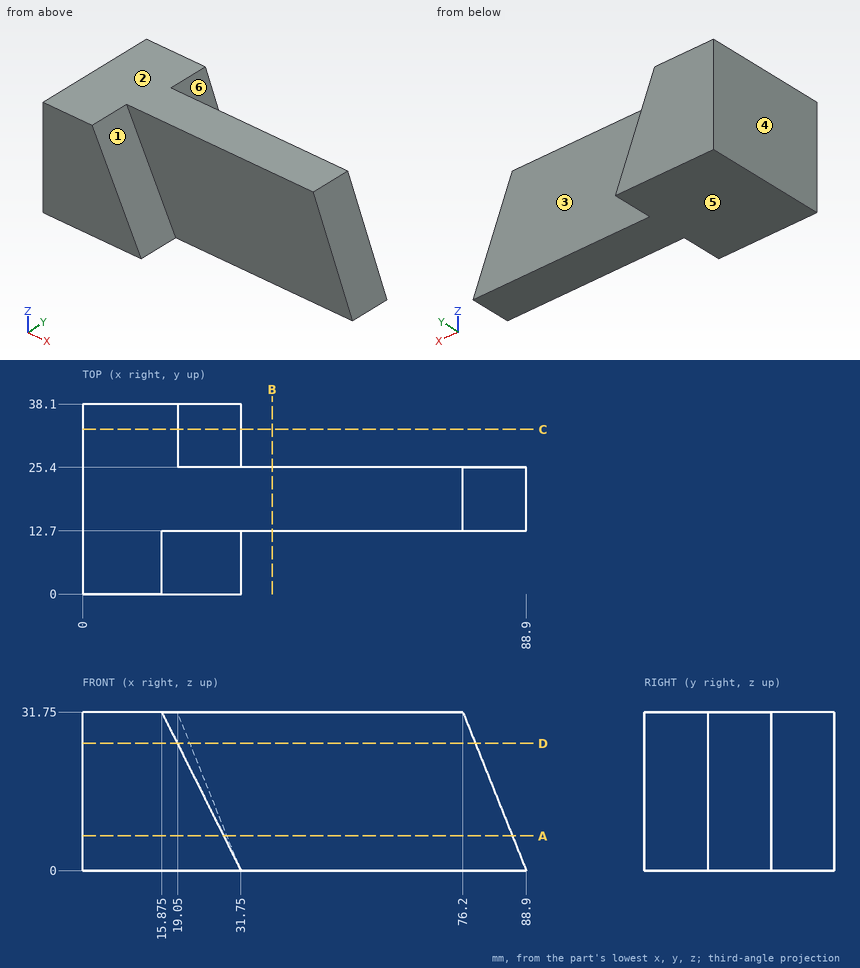
Input: dimensioned drawing with shaded views. Units: mm. Origin: part minimum x, y, z. A direction names the side the tool comes from. Coordinates: 2 decimals unless noted, no trailing zeros. Order: outer loops, then holes, each group sorted by start corner. A loop starts at its lowest first (then second) coordinate and runs counter-clockwise, first axis right, second up. Notation, with made-up numbers: (-14.75, -40) - (18.25, -40) arc R26 ccw to (18.25, -4) - close; hole circle Ø9 at (46, 55.25). An arc over 180 degrees is marked (long way). Return JSON: item names as keys, results as strings. Group by question number.
1. Material intervals for line 1 along Y through (x, z) = (70, 2); line 2 along X through (y, z) = (28.5, 23); line 3 along X through (y, z) = (32, 7), sorted ascending. Write a range as [from, to].
2. Pull-direction query (Z, two-part tool) for the marked faces 4, 5 and 6; classes: pulls with the +Z half, pulls with the -Z half, needs draft (parallel to the pull), parting line crosses it, or undercut.
3. Pin query (flat end, axial travel): pin 1 (9.5 mm diameter, centred on x = 35, z = 18.5, fed in from -Y); pin 2 (9.5 mm diameter, centred on x = 63, z = 20.5, fed in from +Y). Return the tip coordinate at first contact, or that it passes through.
4. Cut plane B-B (x = 38). Output: boundary loops of the cut face in (y, z).
5. Cut plane A-A (z = 7). Output: boundary loops of the cut face in (x, y).
6. Cut plane C-C (y = 33). Output: boundary loops of the cut face in (x, z).
7. Cut plane D-D (z = 25.5). Output: boundary loops of the cut face in (x, y).
8. Set-up query: the marked faces 1, 2 and 3. Return all of +Z, -Z, +X, -X, +Y, -Y with unobstructed straight access to the full face (end or side cutting, diameter ignored); none if empty.
Resolved:
{
 "1": {"line 1": "y = [12.7, 25.4]", "line 2": "x = [0, 22.55]", "line 3": "x = [0, 28.95]"},
 "2": {"face 4": "needs draft", "face 5": "pulls with the -Z half", "face 6": "pulls with the +Z half"},
 "3": {"pin 1": "stops at y = 12.7", "pin 2": "stops at y = 25.4"},
 "4": {"outline": "(12.7, 0) - (25.4, 0) - (25.4, 31.75) - (12.7, 31.75) - close"},
 "5": {"outline": "(0, 0) - (28.25, 0) - (28.25, 12.7) - (86.1, 12.7) - (86.1, 25.4) - (28.95, 25.4) - (28.95, 38.1) - (0, 38.1) - close"},
 "6": {"outline": "(0, 0) - (31.75, 0) - (19.05, 31.75) - (0, 31.75) - close"},
 "7": {"outline": "(0, 0) - (19, 0) - (19, 12.7) - (78.7, 12.7) - (78.7, 25.4) - (21.55, 25.4) - (21.55, 38.1) - (0, 38.1) - close"},
 "8": {"face 1": "+Z, +X, -Y", "face 2": "+Z, +X, -X, +Y, -Y", "face 3": "+Z, +X, +Y"}
}
